from build123d import *

# Parameters (mm, degrees)
SKIZZE1_W                                            = 32
SKIZZE1_H                                            = 26
AUFSATZ_LINEAR_AUSTRAGEN1_DEPTH                      = 2
FORMSENKUNG_F_R_M3_LINSENSENKSCHRAUBE_MI_D           = 3.4
FORMSENKUNG_F_R_M3_LINSENSENKSCHRAUBE_MI_DEPTH       = 8.5
FORMSENKUNG_F_R_M3_LINSENSENKSCHRAUBE_MI_CSINK_D     = 6.3
FORMSENKUNG_F_R_M3_LINSENSENKSCHRAUBE_MI_CSINK_ANGLE = 90
FORMSENKUNG_F_R_M3_LINSENSENKSCHRAUBE_MI_TIP         = 1.021463052
AUFSATZ_LINEAR_AUSTRAGEN2_DEPTH                      = 48
SKIZZE12_W                                           = 27.2
SKIZZE12_H                                           = 16.2
SCHNITT_LINEAR_AUSTRAGEN3_DEPTH                      = 55.083269132
F_3_2_3_2_DURCHMESSER_BOHRUNG1_D                     = 3.2
SKIZZE16_W                                           = 1.1
SKIZZE16_H                                           = 2
SCHNITT_LINEAR_AUSTRAGEN5_DEPTH                      = 55.083269132
VERRUNDUNG1_R                                        = 1


with BuildPart() as part:
    # Skizze1 → Aufsatz-Linear austragen1 (new body)
    with BuildSketch(Plane(origin=(0, 0, 0), x_dir=(1, 0, 0), z_dir=(0, 1, 0))):
        Rectangle(SKIZZE1_W, SKIZZE1_H)
    extrude(amount=AUFSATZ_LINEAR_AUSTRAGEN1_DEPTH)

    # Formsenkung für M3 Linsensenkschraube mit Schlitz1
    with Locations(Plane(origin=(0, 2, 0), x_dir=(1, 0, 0), z_dir=(0, 1, 0))):
        with Locations((-6.5, 9), (3.5, 9)):
            CounterSinkHole(FORMSENKUNG_F_R_M3_LINSENSENKSCHRAUBE_MI_D / 2, FORMSENKUNG_F_R_M3_LINSENSENKSCHRAUBE_MI_CSINK_D / 2, depth=FORMSENKUNG_F_R_M3_LINSENSENKSCHRAUBE_MI_DEPTH, counter_sink_angle=FORMSENKUNG_F_R_M3_LINSENSENKSCHRAUBE_MI_CSINK_ANGLE)
            with Locations((0, 0, -(FORMSENKUNG_F_R_M3_LINSENSENKSCHRAUBE_MI_DEPTH + FORMSENKUNG_F_R_M3_LINSENSENKSCHRAUBE_MI_TIP / 2))):  # 118° drill point
                Cone(0, FORMSENKUNG_F_R_M3_LINSENSENKSCHRAUBE_MI_D / 2, FORMSENKUNG_F_R_M3_LINSENSENKSCHRAUBE_MI_TIP, mode=Mode.SUBTRACT)

    # Skizze11 → Aufsatz-Linear austragen2 (add)
    with BuildSketch(Plane.XZ):
        Polygon((16, 13), (16, -13), (14, -13), (14, -5), (-16, -5), (-16, -3.2), (11.2, -3.2), (11.2, 13), align=None)
    extrude(amount=AUFSATZ_LINEAR_AUSTRAGEN2_DEPTH)

    # Skizze12 → Schnitt-Linear austragen3 (cut, through all)
    with BuildSketch(Plane(origin=(0, 2, 0), x_dir=(1, 0, 0), z_dir=(0, 1, 0))):
        with Locations((-2.4, -4.9)):
            Rectangle(SKIZZE12_W, SKIZZE12_H)
    extrude(amount=-SCHNITT_LINEAR_AUSTRAGEN3_DEPTH, mode=Mode.SUBTRACT)

    # Ø3.2 (3.2) Durchmesser Bohrung1 (through all)
    with Locations(Plane.XY.offset(-3.2)):
        with Locations((-1, -42.5)):
            Hole(F_3_2_3_2_DURCHMESSER_BOHRUNG1_D / 2)

    # Skizze16 → Schnitt-Linear austragen5 (cut, through all)
    with BuildSketch(Plane(origin=(0, 2, 0), x_dir=(1, 0, 0), z_dir=(0, 1, 0))):
        with Locations((11.75, 2.2)):
            Rectangle(SKIZZE16_W, SKIZZE16_H)
    extrude(amount=-SCHNITT_LINEAR_AUSTRAGEN5_DEPTH, mode=Mode.SUBTRACT)

    # Verrundung1
    verrundung1_edges = [part.edges().sort_by_distance(p)[0] for p in [
        (12.3, -23, -3.2),
        (12.3, -23, -1.2),
    ]]
    fillet(verrundung1_edges, radius=VERRUNDUNG1_R - 0.0001)  # a hair under: the kernel refuses the full size


solid = part.part
Part model, mm, in its own coordinate system. A direction names the side the tool comes from. Coordinates: 2 decimals unless noted, no trailing zeros. Order: outer loops, then holes, each group sorted by start corner. A loop starts at its lowest first (then second) coordinate and runs counter-clockwise, first axis right, second up. Notation, with made-up numbers: M 63.25,-13.5 L 115.25,-13.5 A12 cw 115.25,6.5 Z; hole C -29,-36 d11. An arc over 180 degrees is marked long. Use a Markdown table: item, result.
(1) Flat gauge pins, fed straight in: pin 1 (2.5 mm diameter, centred on x = 3.5, z = -9, fed in from -Y); pin 2 (8 mm diameter, centred on x = 2, y = -13.5, fed in from +Z); pin 3 (1.5 mm diameter, centred on x = 10.5, y = -29, fed in from -Z); pin 4 (2.5 mm diameter, centred on y = -34.5, z = -10.5, fed in from -X). Where does each tip first touch, or does it go through?
A:
| item | result |
|---|---|
| pin 1 | passes through |
| pin 2 | stops at z = -3.2 |
| pin 3 | stops at z = -5 |
| pin 4 | stops at x = 14 |
(2) Tool access for faces 1 (the flat face through (11.2, -23, 6)), 2 (the flat face through (-1, -24, -5)), 3 (the cylindrical face through (12.015, -23.35, -2.899)), 4 (the flat face through (14, -23, 13)): list every direction of +Z, -Z, +X, -X, +Y, -Y with a clear straight run to the whole face (end or side of a thin tool).
A:
| item | result |
|---|---|
| face 1 | +Z, -X, +Y, -Y |
| face 2 | -Z, -X, -Y |
| face 3 | -X, +Y, -Y |
| face 4 | +Z, +X, -X, +Y, -Y |
(3) Pull direction X, two halves, no side cores. Call faces 5 (the cylindrical face through (2.7, 0.3, -7.5)), 6 (the flat face through (-16, -19, -4)), 7 (the flat face through (3, 2, -5)): released by +X, released by -X, zero draft, split by the parting line, or undercut.
A:
| item | result |
|---|---|
| face 5 | undercut |
| face 6 | released by -X |
| face 7 | zero draft |
(4) Probe L1, parallel to X at y = 0.25, z = -9; L2, parallel to Z at x = 3.5, y = 0.15; L3, parallel to Y at x = -1, z = -4.3. List the from-to ranges inside material, lowest first.
A:
| item | result |
|---|---|
| L1 | x = -16 to -8.2, -4.8 to 1.8, 5.2 to 16 |
| L2 | z = -13 to -10.7, -7.3 to -3.2 |
| L3 | y = -48 to -44.1, -40.9 to 2 |
(5) Cut at C-C on z = -9. Write the cut outline in (x, y).
A:
| item | result |
|---|---|
| outline | M -16,0 L -8.2,0 L -8.2,0.55 L -9.65,2 L -16,2 Z; M -4.8,0 L 1.8,0 L 1.8,0.55 L 0.35,2 L -3.35,2 L -4.8,0.55 Z; M 5.2,0 L 14,0 L 14,-48 L 16,-48 L 16,2 L 6.65,2 L 5.2,0.55 Z |
(6) Cut at B-B on x = 3.5. Write the cut outline in (y, z), then the cut area to 3 significant figures.
A:
| item | result |
|---|---|
| outline | M -48,-5 L 0,-5 L 0,-7.3 L 0.55,-7.3 L 2,-5.85 L 2,-3.2 L -48,-3.2 Z; M 0,-13 L 2,-13 L 2,-12.15 L 0.55,-10.7 L 0,-10.7 Z |
| area | 97.1 mm^2 |
